Part model, mm, in its own coordinate system. Coordinates: 2 decimals unless noted, no trailing zeros. Write each loop counter-clockwise with the first axis right and the second up, starting at its lowest first coordinate (ties: lowest second). Pieces come first, ordered by that corner, then holes. Notation, with made-up numbers: (-9, 0) - (49, 0) arc R24 ccw to (49, 34) - close; hole circle Ø8 at (53.25, -22.5). An arc over 180 degrees is marked (long way). Use one line per item in the form item = value. Start each with the question number.
from build123d import *

# Parameters (mm, degrees)
F0_R     = 1.5875
F0_R_2   = 0.903846
F1_DEPTH = 88.9
F2_R     = 0.127
F3_DEPTH = 15.24


with BuildPart() as f1:
    # F0 (on Front) → F1 (new body)
    with BuildSketch(Plane.XZ):
        Circle(F0_R)
        Circle(F0_R_2, mode=Mode.SUBTRACT)
    extrude(amount=F1_DEPTH)

    # F2 (on Top) → F3 (join)
    with BuildSketch(Plane.XY):
        with Locations((0, -70.8025)):
            Circle(F2_R)
        with Locations((0, -34.6075)):
            Circle(F2_R)
        with Locations((0, -52.705)):
            Circle(F2_R)
    extrude(amount=F3_DEPTH)


solid = f1.part
Q1. Drill centre lines: probe 1 along Z at (x, y) = (0, -69); probe 2 along Z at (x, y) = (0.75, -66); probe 3 along Z at (x, y) = (-1.05, -70). Where is each one in solid material? Low to high.
Q2. Slice it at B-B (z = 13.5). List the corners of the cut face in (x, y) (1 decimal), plus the area to 3 significant figures.
Q3. Pin check, flat tips, straight feed: P1, Ø1.5, axis at x = -1, z = 4.5, coming from the +Y side; P2, Ø10, axis at y = -47, z = 6, coming from the -X side; P3, Ø1, axis at x = -0.5, z = 10.5, coming from the +Y side; P4, Ø8, axis at y = -23, z = 2.5, coming from the +X side. Stop position of each tip, or through.
Q4. Mould opens along Z. For faces 1 (the cylindrical face through (-0.717, -43.828, -0.55)), 2 (the cylindrical face through (-0.34, -43.83, -1.55)), 3 (the flat face through (1, -88.9, -1)) say: released by +Z, released by -Z, zero draft, split by the parting line, or undercut.
Q5. Slice it at A-A (y = -69). List the corners of the cut face in (x, z) (1 decimal).
Solution:
q1.probe_1 = -1.59 to -0.9, 0.9 to 1.59
q1.probe_2 = -1.4 to -0.5, 0.5 to 1.4
q1.probe_3 = -1.19 to 1.19
q2.outline = circle Ø0.3 at (0, -70.8); circle Ø0.3 at (0, -52.7); circle Ø0.3 at (0, -34.6)
q2.area = 0.152 mm2
q3.P1 = through
q3.P2 = -1.23
q3.P3 = -34.48
q3.P4 = 1.59
q4.face_1 = undercut
q4.face_2 = split by the parting line
q4.face_3 = zero draft
q5.outline = circle Ø3.2 at (0, 0); hole circle Ø1.8 at (0, 0)
